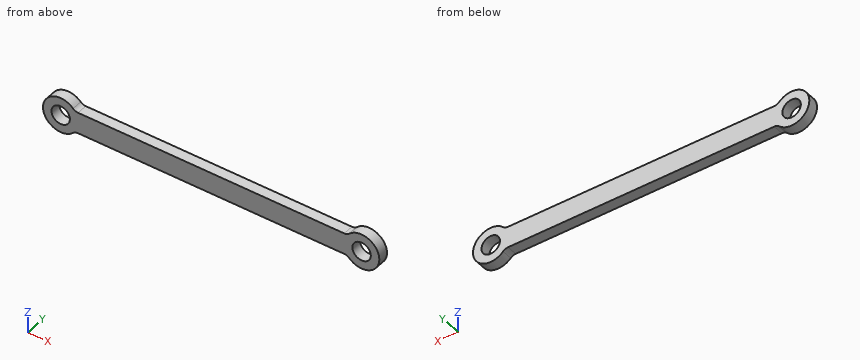
from build123d import *

# Parameters (mm, degrees)
EXTRUDE_1_DEPTH     = 3
SKETCH_2_R          = 5
EXTRUDE_2_DEPTH     = 3
SKETCH_3_R          = 2.6
CUT_EXTRUDE_1_DEPTH = 10
FILLET_1_R          = 2


with BuildPart() as part:
    # ｽｹｯﾁ1 → ﾎﾞｽ - 押し出し1 (new body)
    with BuildSketch(Plane(origin=(0, 0, 0), x_dir=(1, 0, 0), z_dir=(0, 1, 0))):
        with BuildLine():
            Line((-42.5, 3), (42.5, 3))
            ThreePointArc((42.5, 3), (45.5, 0), (42.5, -3))
            Line((42.5, -3), (-42.5, -3))
            ThreePointArc((-42.5, -3), (-45.5, 0), (-42.5, 3))
        make_face()
    extrude(amount=EXTRUDE_1_DEPTH)

    # ｽｹｯﾁ2 → ﾎﾞｽ - 押し出し2 (add)
    with BuildSketch(Plane(origin=(0, 3, 0), x_dir=(1, 0, 0), z_dir=(0, 1, 0))):
        with Locations((-42.5, 0)):
            Circle(SKETCH_2_R)
        with Locations((42.5, 0)):
            Circle(SKETCH_2_R)
    extrude(amount=-EXTRUDE_2_DEPTH)

    # ｽｹｯﾁ3 → ｶｯﾄ - 押し出し1 (cut)
    with BuildSketch(Plane(origin=(0, 3, 0), x_dir=(1, 0, 0), z_dir=(0, 1, 0))):
        with Locations(Location((-42.5, 0, 0), (0, 0, 270))):
            Circle(SKETCH_3_R)
        with Locations(Location((42.5, 0, 0), (0, 0, 270))):
            Circle(SKETCH_3_R)
    extrude(amount=-CUT_EXTRUDE_1_DEPTH, mode=Mode.SUBTRACT)

    # ﾌｨﾚｯﾄ1
    fillet_1_edges = [part.edges().sort_by_distance(p)[0] for p in [
        (-38.5, 1.5, 3),
        (-38.5, 1.5, -3),
        (38.5, 1.5, 3),
        (38.5, 1.5, -3),
    ]]
    fillet(fillet_1_edges, radius=FILLET_1_R)


solid = part.part
Build history of the part. All positions in model axes, mm. Give positions to 0.01 mm unless a question says otherwise; leave off trailing zeros. Order: outer loops, then holes, each group sorted by start corner. A loop starts at its lowest first (then second) coordinate and runs counter-clockwise, first axis right, second up. Notation, with made-up numbers: M -2.75,-5.5 L 1.25,-5.5 A23 ccw 1.25,26.5 Z; hole C 77,71 d5. An arc over 180 degrees is marked long. Put each result on its own line as item: value.
Item 1: Cut at D-D on x = 2.5. Write the cut outline in (y, z), then the cut area to 3 significant figures.
Results are:
outline: M 0,-3 L 3,-3 L 3,3 L 0,3 Z
area: 18.0 mm2
Item 2: Wall check: probe 1 along X at (y, z) = (1.85, 0); probe 2 along Z at (x, y) = (21.5, 0.6); probe 3 along X at (y, z) = (0.5, 3.75). Give the ranges that are in metal, low to high.
Results are:
probe 1: -47.5 to -45.1, -39.9 to 39.9, 45.1 to 47.5
probe 2: -3 to 3
probe 3: -45.81 to -39.19, 39.19 to 45.81
Item 3: Cut at C-C on y = 1.05. Write the cut outline in (x, z).
Results are:
outline: M -39,-3.57 A2 cw -37.6,-3 L 37.6,-3 A2 cw 39,-3.57 A5 ccw long 39,3.57 A2 cw 37.6,3 L -37.6,3 A2 cw -39,3.57 A5 ccw long Z; hole C -42.5,0 d5.2; hole C 42.5,0 d5.2
Item 4: Drop flat-ended pins along their axis: pin 1 Ø1 at (y, z) = (0.5, 1) entering from -X; pin 2 Ø4.5 at (x, z) = (-42.5, 0) entering from +Y; pin 3 Ø0.9 at (x, y) = (2.5, 1) entering from -Z. Give the stop position or say it passes through.
Results are:
pin 1: x = -47.47
pin 2: through
pin 3: z = -3
Item 5: Cut at A-A on x = 42.5. Write the cut outline in (y, z), then the cut area to 3 significant figures.
Results are:
outline: M 0,-5 L 3,-5 L 3,-2.6 L 0,-2.6 Z; M 0,2.6 L 3,2.6 L 3,5 L 0,5 Z
area: 14.4 mm2
Item 6: Cut at B-B on z = 0. Write the cut outline in (x, y).
Results are:
outline: M -47.5,0 L -45.1,0 L -45.1,3 L -47.5,3 Z; M -39.9,0 L 39.9,0 L 39.9,3 L -39.9,3 Z; M 45.1,0 L 47.5,0 L 47.5,3 L 45.1,3 Z
